CAD build for the part. Positions are in the model's coordinates, mm. A direction names the side the tool comes from. Give positions to 0.01 mm unless a question says otherwise; leave off trailing zeros. Write each loop counter-clockwise with the first axis right and the second up, starting at its lowest first coordinate (ties: lowest second). Pieces come first, ordered by that corner, then holes. Notation, with made-up numbers: (40.5, -25.75) -> (61.5, -25.75) arc R35 ccw to (61.5, 6.25) -> close; hole circle Ø5 at (4, -2). An arc over 180 degrees is marked (long way). Answer as a JSON object with one key per item and string values.
```python
from build123d import *

# Parameters (mm, degrees)
PAD003_DEPTH  = 1.6
SKETCH011_W   = 1.3
SKETCH011_H   = 16
PAD004_DEPTH  = 2.25
SKETCH012_W   = 0.8
SKETCH012_H   = 0.65
SKETCH012_W_2 = 0.85
PAD005_DEPTH  = 15


with BuildPart() as part:
    # Sketch008 → Pad003 (new body)
    with BuildSketch(Plane.XY.offset(85)):
        with BuildLine():
            Line((30.57387, -6.02613), (30.57387, -27.02613))
            ThreePointArc((28, -29.6), (29.820001, -28.846131), (30.57387, -27.02613))
            Line((28, -29.6), (-28, -29.6))
            ThreePointArc((-30.57387, -27.02613), (-29.820001, -28.846131), (-28, -29.6))
            Line((-30.57387, -27.02613), (-30.57387, -6.02613))
            ThreePointArc((-30.57387, -6.02613), (-29.827262, -7.828601), (-28.02479, -8.575209))
            Line((-28.02479, -8.575209), (-26.12479, -8.575209))
            Line((-26.12479, -8.575209), (-26.12479, -13.175209))
            Line((-26.12479, -13.175209), (-13.82859, -13.175209))
            Line((-13.82859, -13.175209), (-13.82859, -25.175209))
            Line((-13.82859, -25.175209), (-1.82859, -25.175209))
            Line((-1.82859, -25.175209), (-1.82859, -13.224409))
            Line((-1.82859, -13.224409), (4.37141, -13.224409))
            Line((4.37141, -13.224409), (4.37141, -21.24222))
            Line((4.37141, -21.24222), (16.87141, -21.24222))
            Line((16.87141, -21.24222), (16.87141, -11.37521))
            Line((16.87141, -11.37521), (25.87141, -11.37521))
            Line((25.87141, -11.37521), (25.87141, -8.57521))
            Line((25.87141, -8.57521), (28.02479, -8.57521))
            ThreePointArc((28.02479, -8.57521), (29.827262, -7.828602), (30.57387, -6.02613))
        make_face()
    extrude(amount=PAD003_DEPTH)

    # Sketch011 → Pad004 (new body)
    with BuildSketch(Plane(origin=(0, 0, 85), x_dir=(1, 0, 0), z_dir=(0, 0, -1))):
        with Locations((-28.27479, 16.575209)):
            Rectangle(SKETCH011_W, SKETCH011_H)
        with Locations((28.281635, 16.57521)):
            Rectangle(SKETCH011_W, SKETCH011_H)
    extrude(amount=PAD004_DEPTH)

    # Sketch012 → Pad005 (new body)
    with BuildSketch(Plane(origin=(0, -8.57521, 85), x_dir=(-1, 0, 0), z_dir=(0, 1, 0))):
        with Locations((29.32479, -1.925)):
            Rectangle(SKETCH012_W, SKETCH012_H)
        with Locations((-29.356635, -1.925)):
            Rectangle(SKETCH012_W_2, SKETCH012_H)
    extrude(amount=-PAD005_DEPTH)


solid = part.part
```
1) Slice it at A-A (y = -16). List the corners of the cut face in (x, z), then the cut area to 3 significant figures.
Model answer:
{"outline": "(-30.57, 85) -> (-28.92, 85) -> (-28.92, 83.4) -> (-29.72, 83.4) -> (-29.72, 82.75) -> (-27.62, 82.75) -> (-27.62, 85) -> (-13.83, 85) -> (-13.83, 86.6) -> (-30.57, 86.6) -> close; (-1.83, 85) -> (4.37, 85) -> (4.37, 86.6) -> (-1.83, 86.6) -> close; (16.87, 85) -> (27.63, 85) -> (27.63, 82.75) -> (29.78, 82.75) -> (29.78, 83.4) -> (28.93, 83.4) -> (28.93, 85) -> (30.57, 85) -> (30.57, 86.6) -> (16.87, 86.6) -> close", "area": "65.6 mm2"}
2) 3-axis set-ups, long thin cutter, end or side, ignore diameter. For faces 1 (the flat face through (-20, -13.175, 86)), 2 (the flat face through (-27.625, -16, 84)), 3 (the flat face through (28, -24.575, 84)): which of +Z, -Z, +X, -X, +Y, -Y reach the whole face in a straight line?
Model answer:
{"face 1": "+Z, -Z, +Y", "face 2": "-Z, +Y, -Y", "face 3": "-Z, +X, -X, -Y"}
3) Slice it at D-D (x = -20.5). List the corners of the cut face in (y, z), then the cut area to 3 significant figures.
Model answer:
{"outline": "(-29.6, 85) -> (-13.18, 85) -> (-13.18, 86.6) -> (-29.6, 86.6) -> close", "area": "26.3 mm2"}
4) Slice it at B-B (z = 84.45). List the corners of the cut face in (x, y), then the cut area to 3 significant figures.
Model answer:
{"outline": "(-28.92, -24.58) -> (-27.62, -24.58) -> (-27.62, -8.58) -> (-28.92, -8.58) -> close; (27.63, -24.58) -> (28.93, -24.58) -> (28.93, -8.58) -> (27.63, -8.58) -> close", "area": "41.6 mm2"}
5) Slice it at C-C (x = -27). List the corners of the cut face in (y, z), then the cut area to 3 significant figures.
Model answer:
{"outline": "(-29.6, 85) -> (-8.58, 85) -> (-8.58, 86.6) -> (-29.6, 86.6) -> close", "area": "33.6 mm2"}
6) Wall check: probe 1 along X at (y, z) = (-14.5, 86.3); probe 2 along X at (y, z) = (-11.75, 84.6); probe 3 along X at (y, z) = (-12, 86.2). Give the ranges that are in metal, low to high.
Model answer:
{"probe 1": "x = -30.57 to -13.83, -1.83 to 4.37, 16.87 to 30.57", "probe 2": "x = -28.92 to -27.62, 27.63 to 28.93", "probe 3": "x = -30.57 to -26.12, 16.87 to 30.57"}
7) Pin check, flat tips, straight feed: pin 1 (1.8 mm diameter, centred on x = 8.5, z = 85.5, fed in from +Y); pin 2 (0.5 mm diameter, centred on x = -29, z = 83, fed in from +Y); pin 3 (0.8 mm diameter, centred on x = -18, z = 85.5, fed in from +Y). Stop position of each tip, or through.
Model answer:
{"pin 1": "stops at y = -21.24", "pin 2": "stops at y = -8.58", "pin 3": "stops at y = -13.18"}
8) Mould opens along X. For faces 4 (the cylindrical face through (29.8, -28.866, 85.789)), 5 (the flat face through (-28, -24.575, 84)), 6 (the flat face through (27.9, -8.575, 84.7)) say: released by +X, released by -X, zero draft, split by the parting line, or undercut.
Model answer:
{"face 4": "released by +X", "face 5": "zero draft", "face 6": "undercut"}
